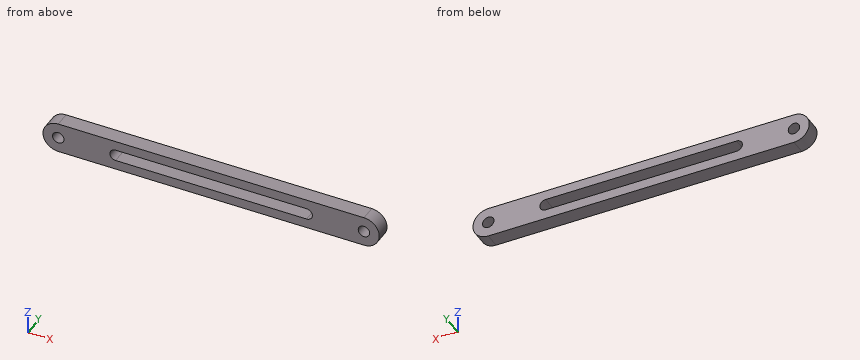
```python
from build123d import *

# Parameters (mm, degrees)
F0_R     = 1.5
F1_DEPTH = 2
F3_DEPTH = 25


with BuildPart() as f1:
    # F0 (on Front) → F1 (new body, symmetric)
    with BuildSketch(Plane.XZ):
        with BuildLine():
            ThreePointArc((40, -4), (44, 0), (40, 4))
            Line((40, 4), (-40, 4))
            ThreePointArc((-40, 4), (-44, 0), (-40, -4))
            Line((-40, -4), (40, -4))
        make_face()
        with Locations((-40, 0)):
            Circle(F0_R, mode=Mode.SUBTRACT)
        with Locations((-10, 0)):
            Circle(F0_R, mode=Mode.SUBTRACT)
        with Locations((40, 0)):
            Circle(F0_R, mode=Mode.SUBTRACT)
    extrude(amount=F1_DEPTH, both=True)

    # F2 (on face) → F3 (cut)
    with BuildSketch(Plane.XZ.offset(2)):
        with BuildLine():
            Line((-10, 1.5), (-25, 1.5))
            ThreePointArc((-25, 1.5), (-26.5, 0), (-25, -1.5))
            Line((-25, -1.5), (-10, -1.5))
            ThreePointArc((-10, -1.5), (-11.5, 0), (-10, 1.5))
        make_face()
        with BuildLine():
            Line((25, 1.5), (-10, 1.5))
            ThreePointArc((-10, 1.5), (-8.93934, 1.06066), (-8.5, 0))
            ThreePointArc((-8.5, 0), (-8.93934, -1.06066), (-10, -1.5))
            Line((-10, -1.5), (25, -1.5))
            ThreePointArc((25, -1.5), (26.5, 0), (25, 1.5))
        make_face()
    extrude(amount=-F3_DEPTH, mode=Mode.SUBTRACT)


solid = f1.part
```
Verification items for the finished model (mm, model axes). Give positions to 0.01 mm unless a question says otherwise; leave off trailing zeros. Order: outer loops, then holes, each group sorted by start corner. A loop starts at its lowest first (then second) coordinate and runs counter-clockwise, first axis right, second up. Notation, with made-up numbers: (-39.75, 68) -> (-22.75, 68) arc R19 cw to (-22.75, 100) -> close; hole circle Ø10 at (60.5, 30.25). An arc over 180 degrees is marked (long way). Use a Markdown table: item, result.
1) Section check A-A, the plane x = 19.5. Record the boundary of the cut face in (y, z).
Results:
| item | result |
|---|---|
| outline | (-2, -4) -> (2, -4) -> (2, -1.5) -> (-2, -1.5) -> close; (-2, 1.5) -> (2, 1.5) -> (2, 4) -> (-2, 4) -> close |
2) Depth check by flat-ended pin: pin 1 Ø1 at (y, z) = (-0.5, -2.5) entering from -X. Enter the tip coordinate at first touch or a pass-through.
Results:
| item | result |
|---|---|
| pin 1 | x = -43.46 |
3) Material ranges on probe 1 along Z at (x, y) = (-12.5, -1.6); probe 2 along X at (y, z) = (-0.75, -1.25); probe 3 along X at (y, z) = (0.9, 0.25), recorded low to high.
Results:
| item | result |
|---|---|
| probe 1 | -4 to -1.5, 1.5 to 4 |
| probe 2 | -43.8 to -40.83, -39.17 to -25.83, 25.83 to 39.17, 40.83 to 43.8 |
| probe 3 | -43.99 to -41.48, -38.52 to -26.48, 26.48 to 38.52, 41.48 to 43.99 |
4) Section check C-C, the plane z = 0. Record the boundary of the cut face in (x, y), then the cut area to 3 significant figures.
Results:
| item | result |
|---|---|
| outline | (-44, -2) -> (-41.5, -2) -> (-41.5, 2) -> (-44, 2) -> close; (-38.5, -2) -> (-26.5, -2) -> (-26.5, 2) -> (-38.5, 2) -> close; (26.5, -2) -> (38.5, -2) -> (38.5, 2) -> (26.5, 2) -> close; (41.5, -2) -> (44, -2) -> (44, 2) -> (41.5, 2) -> close |
| area | 116 mm² |
5) Section check B-B, the plane y = 1.35. Record the boundary of the cut face in (x, z), then the cut area to 3 significant figures.
Results:
| item | result |
|---|---|
| outline | (-40, -4) -> (40, -4) arc R4 ccw to (40, 4) -> (-40, 4) arc R4 ccw to start; hole circle Ø3 at (-40, 0); hole (-25, -1.5) -> (25, -1.5) arc R1.5 ccw to (25, 1.5) -> (-25, 1.5) arc R1.5 ccw to start; hole circle Ø3 at (40, 0) |
| area | 519 mm² |
